```python
from build123d import *

# Parameters (mm, degrees)
F1_R     = 10.75
F2_DEPTH = 5
F3_DEPTH = 1
F0_W     = 1.6666666667
F0_H     = 1.6666666667
F4_DEPTH = 12.5


with BuildPart() as f2:
    # F1 (on Top) → F2 (new body)
    with BuildSketch(Plane.XY):
        Circle(F1_R)
        with BuildLine():
            ThreePointArc((-8.6602540538, 4.9999999724), (-5.0000000138, 8.6602540299), (0, 10))
            ThreePointArc((0, 10), (5.0000000138, 8.6602540299), (8.6602540538, 4.9999999724))
            ThreePointArc((8.6602540538, 4.9999999724), (9.659258267, 2.5881904356), (10, 0))
            ThreePointArc((10, 0), (9.6592582663, -2.5881904384), (8.6602540509, -4.9999999774))
            ThreePointArc((8.6602540509, -4.9999999774), (5.0000000086, -8.6602540329), (-6.2e-09, -10))
            ThreePointArc((-6.2e-09, -10), (-5.0000000165, -8.6602540283), (-8.6602540538, -4.9999999724))
            ThreePointArc((-8.6602540538, -4.9999999724), (-10, 0), (-8.6602540538, 4.9999999724))
        make_face(mode=Mode.SUBTRACT)
        with BuildLine():
            ThreePointArc((8.6602540538, 4.9999999724), (5.0000000138, 8.6602540299), (0, 10))
            ThreePointArc((0, 10), (-5.0000000138, 8.6602540299), (-8.6602540538, 4.9999999724))
            ThreePointArc((-8.6602540538, 4.9999999724), (-10, 0), (-8.6602540538, -4.9999999724))
            ThreePointArc((-8.6602540538, -4.9999999724), (-5.0000000165, -8.6602540283), (-6.2e-09, -10))
            ThreePointArc((-6.2e-09, -10), (5.0000000086, -8.6602540329), (8.6602540509, -4.9999999774))
            ThreePointArc((8.6602540509, -4.9999999774), (9.6592582663, -2.5881904384), (10, 0))
            ThreePointArc((10, 0), (9.659258267, 2.5881904356), (8.6602540538, 4.9999999724))
        make_face()
        with BuildLine():
            ThreePointArc((-5.3947095812, -4.125), (-6.6917762677, -5.8153702001), (-8.6602540538, -4.9999999724))
            ThreePointArc((-8.6602540538, -4.9999999724), (-7.5976428947, -2.4346297999), (-5.3947095812, -4.125))
        make_face(mode=Mode.SUBTRACT)
        with BuildLine():
            ThreePointArc((1.75, -8.25), (1.2374368649, -9.4874368693), (-6.2e-09, -10))
            ThreePointArc((-6.2e-09, -10), (-1.2374368649, -7.0125631307), (1.75, -8.25))
        make_face(mode=Mode.SUBTRACT)
        with BuildLine():
            ThreePointArc((8.8947095812, -4.125), (8.8350797806, -4.5779333163), (8.6602540509, -4.9999999774))
            ThreePointArc((8.6602540509, -4.9999999774), (5.4543393818, -3.6720666837), (8.8947095812, -4.125))
        make_face(mode=Mode.SUBTRACT)
        with BuildLine():
            ThreePointArc((-5.3947095812, 4.125), (-7.5976428947, 2.4346297999), (-8.6602540538, 4.9999999724))
            ThreePointArc((-8.6602540538, 4.9999999724), (-6.6917762677, 5.8153702001), (-5.3947095812, 4.125))
        make_face(mode=Mode.SUBTRACT)
        with BuildLine():
            ThreePointArc((1.75, 5.7391201416), (4.8218253805, 3.5707142143), (6, 0))
            ThreePointArc((6, 0), (-3.5707142143, -4.8218253805), (-1.75, 5.7391201416))
            Line((-1.75, 5.7391201416), (-1.75, 8))
            Line((-1.75, 8), (-1.7320508076, 8))
            ThreePointArc((-1.7320508076, 8), (-1.3228756555, 9.3956439237), (0, 10))
            ThreePointArc((0, 10), (1.2374368671, 9.4874368671), (1.75, 8.25))
            ThreePointArc((1.75, 8.25), (1.745506934, 8.1246782406), (1.7320508076, 8))
            Line((1.7320508076, 8), (1.75, 8))
            Line((1.75, 8), (1.75, 5.7391201416))
        make_face(mode=Mode.SUBTRACT)
        with BuildLine():
            ThreePointArc((8.8947095812, 4.125), (5.4543393811, 3.6720666865), (8.6602540538, 4.9999999724))
            ThreePointArc((8.6602540538, 4.9999999724), (8.8350797814, 4.5779333135), (8.8947095812, 4.125))
        make_face(mode=Mode.SUBTRACT)
    extrude(amount=F2_DEPTH)

    # F1 (on Top) → F3 (join)
    with BuildSketch(Plane.XY):
        with BuildLine():
            ThreePointArc((-1.75, 5.7391201416), (-3.5707142143, -4.8218253805), (6, 0))
            ThreePointArc((6, 0), (4.8218253805, 3.5707142143), (1.75, 5.7391201416))
            ThreePointArc((1.75, 5.7391201416), (0, 6), (-1.75, 5.7391201416))
        make_face()
    extrude(amount=F3_DEPTH)

    # F0 (on Top) → F4 (cut, symmetric)
    with BuildSketch(Plane.XY):
        with Locations((0, 1.6666666667)):
            Rectangle(F0_W, F0_H)
        Rectangle(F0_W, F0_H)
        with Locations((-1.6666666667, 0)):
            Rectangle(F0_W, F0_H)
        with Locations((1.6666666667, 0)):
            Rectangle(F0_W, F0_H)
        with Locations((0, -1.6666666667)):
            Rectangle(F0_W, F0_H)
    extrude(amount=F4_DEPTH, both=True, mode=Mode.SUBTRACT)


solid = f2.part
```
For this review, take the finished solid that the model builds, in its own axes (mm). A direction names the side the tool comes from. Round coordinates to 2 decimals unless told otherwise and drop trailing zeros. Loops run counter-clockwise (first coordinate to the right, second up) from the corner with the lowest first, then second, coordinate; pieces in that order, holes last.
Q1. Add section A-A on z = 1.45. Write out the cut boundary in (x, y) (3 decimals), plus the area to 3 significant figures.
Result sheet:
outline: circle Ø21.5 at (0, 0); hole circle Ø3.5 at (-7.145, -4.125); hole circle Ø3.5 at (-7.145, 4.125); hole circle Ø3.5 at (0, -8.25); hole (-1.75, 5.739) arc R6 ccw (long way) to (1.75, 5.739) - (1.75, 8) - (1.732, 8) arc R1.75 ccw (long way) to (-1.732, 8) - (-1.75, 8) - close; hole circle Ø3.5 at (7.145, -4.125); hole circle Ø3.5 at (7.145, 4.125)
area: 189 mm2
Q2. Insertion check: pin 1 Ø3.5 at (x, y) = (-1, 2) entering from +Z; pin 2 Ø2.5 at (y, z) = (6.5, 3.5) entering from -X; pin 3 Ø1 at (y, z) = (-5, 2) entering from +X; pin 4 Ø1.5 at (x, y) = (2, 7.5) entering from -Z. Each pin has a flat end and moves straight along its axis. Give the tip position at first contact, or say it passes through.
Result sheet:
pin 1: stops at z = 1
pin 2: stops at x = -9.38
pin 3: stops at x = 9.76
pin 4: stops at z = 0
Q3. To check wall thickness, follow line 1 along Y through (x, z) = (-1, 2.7); line 2 along Y through (x, z) = (-8, 2.45); line 3 along Y through (x, z) = (-1.25, 0.6). State the ranges of each line that lie inside material, in increasing order.
Result sheet:
line 1: y = -10.7 to -9.69, -6.81 to -5.92, 9.69 to 10.7
line 2: y = -7.18 to -5.65, -2.6 to 2.6, 5.65 to 7.18
line 3: y = -10.68 to -9.47, -7.03 to -0.83, 0.83 to 5.87, 9.47 to 10.68
Q4. Mouldability with a two-part tool opening along Y and no side actions: class faces 4 (the face through (-2.5, 0, 0.5)), 5 (the face through (-3, 0, 0)), 6 (the face through (-1.4, 10.66, 2.46)), 7 (the face through (1.7, -0.833, 0.5)) as +Y half, -Y half, draft (parallel to the pull), parting line (faces both ways), or undercut.
Result sheet:
face 4: undercut
face 5: draft
face 6: parting line
face 7: undercut
Q5. Add section B-B on y = -7. Write out the cut boundary in (x, z).
Result sheet:
outline: (-8.16, 0) - (-1.22, 0) - (-1.22, 5) - (-8.16, 5) - close; (1.22, 0) - (8.16, 0) - (8.16, 5) - (1.22, 5) - close
Q6. Machinability: for faces 1 (the face through (-1.75, 7, 2)), 2 (the face through (1, -1, 1)), 3 (the face through (5, -5, 5)), which of the approach directions +Z, -Z, +X, -X, +Y, -Y give a long, thin tool a straight path to every point of the face, cutting with its end or side? Answer none if there is none.
Result sheet:
face 1: +Z, -Z
face 2: +Z
face 3: +Z, +X, -X, +Y, -Y
